from build123d import *

# Parameters (mm, degrees)
F0_W     = 12.7625
F0_H     = 20.7
F0_R     = 1.35255
F0_R_2   = 4
F1_DEPTH = 6.35
F2_SIZE  = 0.254


# Not quite as in the source:
# - a feature names something its author has since deleted; it is built from what else it names


with BuildPart() as f1:
    # F0 (on Top) → F1 (new body)
    with BuildSketch(Plane.XY):
        Rectangle(F0_W, F0_H)
        with Locations((0, -7.175)):
            Circle(F0_R, mode=Mode.SUBTRACT)
        Circle(F0_R_2, mode=Mode.SUBTRACT)
        with Locations((0, 7.175)):
            Circle(F0_R, mode=Mode.SUBTRACT)
    extrude(amount=F1_DEPTH)

    # F2
    f2_edges = [f1.edges().sort_by_distance(p)[0] for p in [
        (-4, 0, 6.35),
    ]]
    chamfer(f2_edges, length=F2_SIZE)


solid = f1.part
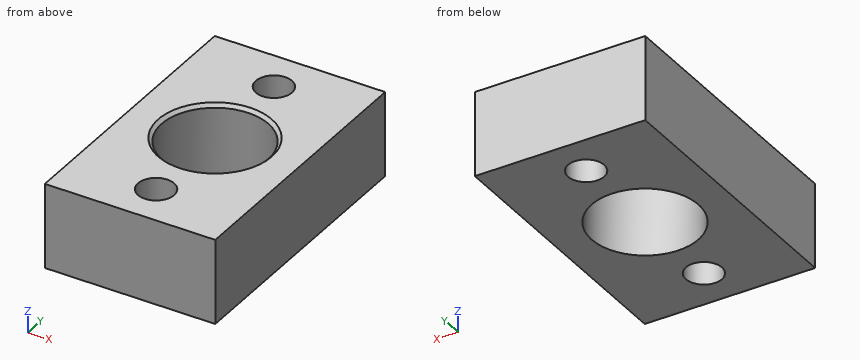
Model file for the job. Use its own axes, mm. Give positions to 0.01 mm unless a question says otherwise; leave off trailing zeros. Loops run counter-clockwise (first coordinate to the right, second up) from the corner with the lowest first, then second, coordinate; pieces in that order, holes last.
Item 1: Slice it at D-D (y = 7.5). Write the cut outline in (x, z).
Check values:
outline: (-6.38, 0) - (-1.31, 0) - (-1.31, 6.35) - (-6.38, 6.35) - close; (1.31, 0) - (6.38, 0) - (6.38, 6.35) - (1.31, 6.35) - close
Item 2: Slice it at C-C (z = 3.75). Write the cut outline in (x, y) (3 decimals), plus the area to 3 significant figures.
Check values:
outline: (-6.381, -10.35) - (6.381, -10.35) - (6.381, 10.35) - (-6.381, 10.35) - close; hole circle Ø8 at (0, 0); hole circle Ø2.705 at (0, -7.175); hole circle Ø2.705 at (0, 7.175)
area: 202 mm2
Item 3: Slice it at B-B (y = 0). Write the cut outline in (x, z).
Check values:
outline: (-6.38, 0) - (-4, 0) - (-4, 6.1) - (-4.25, 6.35) - (-6.38, 6.35) - close; (4, 0) - (6.38, 0) - (6.38, 6.35) - (4.25, 6.35) - (4, 6.1) - close
Item 4: Drill centre lines: line 1 along Y through (x, z) = (0, 1.5); line 2 along X through (y, z) = (-2.25, 4.25); line 3 along Y through (x, z) = (0.5, 4.5). Where is each one in solid material? Low to high.
Check values:
line 1: y = -10.35 to -8.53, -5.82 to -4, 4 to 5.82, 8.53 to 10.35
line 2: x = -6.38 to -3.31, 3.31 to 6.38
line 3: y = -10.35 to -8.43, -5.92 to -3.97, 3.97 to 5.92, 8.43 to 10.35
Item 5: Slice it at A-A (x = 0). Write the cut outline in (y, z), plus the area to 3 significant figures.
Check values:
outline: (-10.35, 0) - (-8.53, 0) - (-8.53, 6.35) - (-10.35, 6.35) - close; (-5.82, 0) - (-4, 0) - (-4, 6.1) - (-4.25, 6.35) - (-5.82, 6.35) - close; (4, 0) - (5.82, 0) - (5.82, 6.35) - (4.25, 6.35) - (4, 6.1) - close; (8.53, 0) - (10.35, 0) - (10.35, 6.35) - (8.53, 6.35) - close
area: 46.2 mm2
Item 6: Drop a flat-ended pin along its axis: P1, Ø5, axis at x = 4, y = 8, coming from the -Z side. Give the stop position or say it passes through.
Check values:
P1: stops at z = 0
